Solid Edge part; units mm, degrees
sketch "Sketch1" plane through (0, 13.8, 0) normal (0, 1, 0) x (-1, 0, 0)
  line L0 (-22.5, 20) -> (-22.5, -20)
  line L1 (-22.5, -20) -> (-22.5, -28)
  line L2 (-22.5, -28) -> (22.5, -28)
  line L3 (22.5, -28) -> (22.5, -20)
  line L4 (22.5, -20) -> (22.5, 20)
  line L5 (22.5, 20) -> (-22.5, 20)
  circle A0 centre (-15, 9) radius 2.5
  circle A1 centre (15, 9) radius 2.5
extrude "ExtrudedProtrusion_1" add sketch "Sketch1" along normal blind 7
mirror "Mirror1" about plane through (0, 0, 0) normal (0, -1, 0) of "ExtrudedProtrusion_1"
sketch "Sketch2" plane through (0, 20.8, -4) normal (0, 1, 0) x (-1, 0, 0)
  line L0 (-22.5, -24) -> (22.5, -24)
  line L1 (22.5, -24) -> (22.5, -31)
  line L2 (22.5, -31) -> (-22.5, -31)
  line L3 (-22.5, -31) -> (-22.5, -24)
extrude "ExtrudedProtrusion_3" add sketch "Sketch2" against normal blind 41.6
sketch "Sketch3" plane through (0, 0, -35) normal (0, 0, -1) x (1, 0, 0)
  circle A0 centre (0, 0) radius 2.5
extrude "ExtrudedCutout_1" cut sketch "Sketch3" against normal blind 32
fillet "Round_2" radius 3 4 edges at (22.5, -17.3, 20) (-22.5, -17.3, 20) (22.5, 17.3, 20) (-22.5, 17.3, 20)
sketch "Sketch4" plane through (0, -20.8, -7.5) normal (0, -1, 0) x (-1, 0, 0)
  line L0 (-22.5, 27.5) -> (22.5, 27.5)
  line L1 (22.5, 27.5) -> (22.5, 22.5)
  line L2 (22.5, 22.5) -> (-22.5, 22.5)
  line L3 (-22.5, 22.5) -> (-22.5, 27.5)
extrude "ExtrudedProtrusion_4" add sketch "Sketch4" along normal blind 45
sketch "Sketch5" plane through (0, -43.3, -30) normal (0, 0, 1) x (0, -1, 0)
  circle A0 centre (0, 0) radius 10.5
  circle A1 centre (-15.5, 15.5) radius 1.5
  circle A2 centre (15.5, 15.5) radius 1.5
  circle A3 centre (15.5, -15.5) radius 1.5
  circle A4 centre (-15.5, -15.5) radius 1.5
extrude "ExtrudedCutout_2" cut sketch "Sketch5" against normal blind 29.9875
fillet "Round_3" radius 1 2 edges at (0, -65.8, -30) (0, -65.8, -35)
sketch "Sketch6" plane through (0, -22, -35) normal (0, 0, -1) x (0, -1, 0)
  circle A0 centre (-22, 0) radius 11
extrude "ExtrudedCutout_3" cut sketch "Sketch6" against normal blind 4
sketch "Sketch7" plane through (0, 0, -31) normal (0, 0, -1) x (0, -1, 0)
  circle A0 centre (0, 0) radius 9
extrude "ExtrudedCutout_4" cut sketch "Sketch7" against normal blind 20
sketch "Sketch8" plane through (0, -22, -35) normal (0, 0, -1) x (1, 0, 0)
  circle A0 centre (0, -4.04) radius 1.5
  circle A1 centre (-15.5538, -30.98) radius 1.5
  circle A2 centre (15.5538, -30.98) radius 1.5
extrude "ExtrudedCutout_5" cut sketch "Sketch8" against normal blind 15
sketch "Sketch9" plane through (0, -20.8, -5) normal (0, -1, 0) x (1, 0, 0)
  line L0 (4, -23) -> (4, -18)
  line L1 (4, -18) -> (-4, -18)
  line L2 (-4, -18) -> (-4, -23)
  line L3 (-4, -23) -> (4, -23)
extrude "ExtrudedCutout_6" cut sketch "Sketch9" against normal blind 10
sketch "Sketch10" plane through (0, -22, -35) normal (0, 0, -1) x (0, 1, 0)
  circle A0 centre (22, 0) radius 11
  circle A1 centre (22, 0) radius 13
extrude "ExtrudedProtrusion_5" add sketch "Sketch10" along normal blind 2.5
fillet "Round_4" radius 1 1 edges at (0, -13, -35)
sketch "Sketch11" plane through (-22.5, -22.5, -9) normal (-1, 0, 0) x (0, 1, 0)
  line L0 (1.7, 6) -> (-13.3, 21)
  line L1 (-13.3, 21) -> (-13.3, 26)
  line L2 (-13.3, 26) -> (8.7, 26)
  line L3 (8.7, 26) -> (8.7, 6)
  line L4 (1.7, 6) -> (8.7, 6)
extrude "ExtrudedProtrusion_6" add sketch "Sketch11" along normal blind 3
chamfer "Chamfer_1" distance 3 angle 45 1 edges at (-22.5, -17.3, -15) measured on face at (-24.97, -19.7033, -15)
chamfer "Chamfer_2" distance 3 angle 45 1 edges at (-22.5, -35.8, -32.5) measured on face at (-24.97, -35.8, -30.7833)
Work out the finished part from the listing and answer in its coordinate system (mm). A direction names the side the tool comes from. Give positions to 0.01 mm unless a question says otherwise; leave off trailing zeros. Order: outer loops, then holes, each group sorted by start corner. A loop starts at its lowest first (then second) coordinate and runs counter-clockwise, first axis right, second up.
1. Straight lines are drawn through the part: L1, parallel to X at y = -58.8, z = -32.4; L2, parallel to Y at x = -19, z = -15; L3, parallel to X at y = 0, z = -30. For each, find the intervals that lie inside material, in ascending order.
Result sheet:
L1: x = -22.5 to -17, -14 to 14, 17 to 22.5
L2: y = -20.8 to -13.8, 13.8 to 20.8
L3: x = -22.5 to -9, 9 to 22.5
2. Section C-C, the plane y = -27.8 is taken. Determine the outline of the cut face in (x, z), and give its area (3 significant figures).
Result sheet:
outline: (-25.5, -35) - (-17, -35) - (-17, -30) - (-22.5, -30) - (-22.5, -22) - (-25.5, -22) - close; (-14, -35) - (14, -35) - (14, -30) - (-14, -30) - close; (17, -35) - (22.5, -35) - (22.5, -30) - (17, -30) - close
area: 234 mm2
3. Each of these flat-tipped pins is pushed along its axis until it touches: P1, Ø3.5, axis at x = -2, y = -17.5, coming from the -Z side; P2, Ø7.5, axis at y = -16, z = -4, coming from the -X side; P3, Ø12, axis at y = -37.5, z = -31.5, coming from the -X side; P4, Ø1.8, axis at x = 0, y = -17.96, coming from the -Z side. Where does it stop, or does it pass through?
Result sheet:
P1: stops at z = -35
P2: stops at x = -22.5
P3: stops at x = -25.5
P4: stops at z = -20
4. Section A-A, the plane z = -6.5 is taken. Determine the outline of the cut face in (x, y).
Result sheet:
outline: (-22.5, -20.8) - (22.5, -20.8) - (22.5, -13.8) - (-22.5, -13.8) - close; (-22.5, 13.8) - (22.5, 13.8) - (22.5, 20.8) - (-22.5, 20.8) - close
5. Section D-D, the plane y = -17.96 is taken. Determine the outline of the cut face in (x, z).
Result sheet:
outline: (-25.5, -35) - (-1.5, -35) - (-1.5, -28) - (-4, -28) - (-4, -23) - (-1.5, -23) - (-1.5, -20) - (1.5, -20) - (1.5, -23) - (4, -23) - (4, -28) - (1.5, -28) - (1.5, -35) - (22.5, -35) - (22.5, 17) arc R3 ccw to (19.5, 20) - (-19.5, 20) arc R3 ccw to (-22.5, 17) - (-22.5, -12) - (-25.5, -15) - close; hole circle Ø5 at (-15, 9); hole circle Ø5 at (15, 9)
6. The mould has two halves that part along Y. Classify faces 1 (the flat face through (-22.5, 15, -19)), 2 (the cylindrical face through (-8.923, 1.172, -29.521)), 3 (the flat face through (0, -65.8, -33)): released by +Y, released by -Y, zero draft, split by the parting line, or undercut.
Result sheet:
face 1: zero draft
face 2: undercut
face 3: released by -Y
7. For faces 4 (the flat face through (11, 3, -37.5)), 5 (the flat face through (-1, -20.8, -5)), 6 (the flat face through (-2, -9, -31)), determine the directions among +Z, -Z, +X, -X, +Y, -Y from which every point of the face is accessible in a straight line to the end or side of a thin tool.
Result sheet:
face 4: -Z, +X, -X, +Y, -Y
face 5: +Z, +X, -Y
face 6: -Z
8. Section B-B, the plane y = 0 is taken. Determine the outline of the cut face in (x, z), and give its area (3 significant figures).
Result sheet:
outline: (-22.5, -35) - (-14, -35) arc R1 cw to (-13, -36) - (-13, -37.5) - (-11, -37.5) - (-11, -31) - (-9, -31) - (-9, -28) - (-22.5, -28) - close; (9, -31) - (11, -31) - (11, -37.5) - (13, -37.5) - (13, -36) arc R1 cw to (14, -35) - (22.5, -35) - (22.5, -28) - (9, -28) - close
area: 183 mm2
